Job drawing, mm, ordinate dimensions from the low corner. One solid piece. A direction names the side the tool comes from. Round coordinates to 2 decimals unless told otherwise and drop trailing zeros. Order: outer loops, then holes, each group sorted by start corner. A loop starts at its lowest first (then second) coordinate and runs counter-clockwise, first axis right, second up. Notation, with made-up numbers: (-24.75, 74) -> (-15.75, 74) arc R10 ccw to (-15.75, 92) -> close; hole circle Ø7 at (33.5, 27). An arc over 180 degrees is marked (long way). Use CSV: the item, a comma, the result in double quotes.
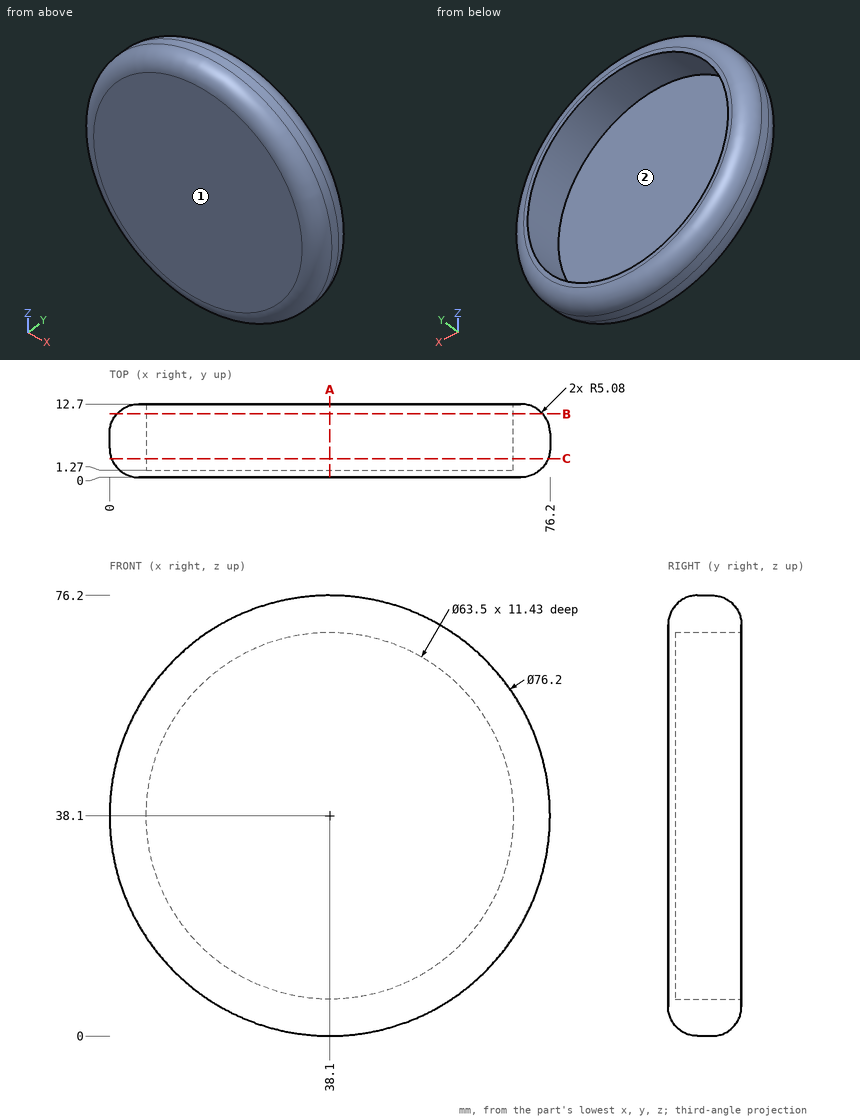
(1) Drop flat-ended pins along their axis: P1, Ø4, axis at x = 22, y = 7.5, coming from the +Z side; P2, Ø1.5, axis at x = 33.5, y = 1.5, coming from the -Z side; P3, Ø3, axis at y = 10, z = 53.5, coming from the -X side; P4, Ø10, axis at x = 21, z = 30.5, coming from the -Y side. Give the stop position or say it passes through.
Reply:
P1,"z = 73.49"
P2,"z = 1.14"
P3,"x = 2.98"
P4,"y = 0"
(2) Cut at A-A, the plane x = 38.1. Give the cut face in (y, z).
Reply:
outline,"(0, 5.08) arc R5.08 ccw to (5.08, 0) -> (7.62, 0) arc R5.08 ccw to (12.7, 5.08) -> (12.7, 6.35) -> (1.27, 6.35) -> (1.27, 69.85) -> (12.7, 69.85) -> (12.7, 71.12) arc R5.08 ccw to (7.62, 76.2) -> (5.08, 76.2) arc R5.08 ccw to (0, 71.12) -> close"
(3) Which spindle directions (+Z, -Z, +X, -X, +Y, -Y) get a long thin tool onto all of the face, cutting with end or side? Do the marked faces 1 and 2. Say none if no direction does.
Reply:
face 1,"+Z, -Z, +X, -X, -Y"
face 2,"+Y"
(4) Cut at C-C, the plane y = 3.25. Give the cut face in (x, z).
Reply:
outline,"circle Ø75.52 at (38.1, 38.1); hole circle Ø63.5 at (38.1, 38.1)"
(5) Probe probe 1 along Y at (x, z) = (34.5, 22.5); probe 2 along Z at (x, y) = (38.1, 6.5); probe 3 along Z at (x, y) = (48, 6). List the from-to ranges inside material, lowest first. Write a range as [from, to].
Reply:
probe 1,"[0, 1.27]"
probe 2,"[0, 6.35], [69.85, 76.2]"
probe 3,"[1.31, 7.93], [68.27, 74.89]"
(6) Cut at B-B, the plane y = 11. Give the cut face in (x, z), then the cut area to 3 significant figures.
Reply:
outline,"circle Ø73.62 at (38.1, 38.1); hole circle Ø63.5 at (38.1, 38.1)"
area,"1,090 mm2"
